Here's how the part is built. I have some questions about the finished solid (model axes, mm). A direction names the side the tool comes from. Round coordinates to 2 decimals unless told otherwise and drop trailing zeros. Order: outer loops, then holes, each group sorted by start corner. A loop starts at its lowest first (then second) coordinate and runs counter-clockwise, first axis right, second up. Notation, with made-up numbers: (22.25, 31) -> (39.25, 31) arc R13 ccw to (39.25, 52) -> close; hole circle Ø8 at (-20.75, 19.5). An arc over 180 degrees is marked (long way). Use a Markdown table: item, result. Add a question column.
from build123d import *

# Parameters (mm, degrees)
F0_W     = 60
F0_H     = 120
F1_DEPTH = 60
F2_R     = 3
F3_DEPTH = 7
F4_R     = 20
F5_R     = 10
F6_R     = 23.5
F7_DEPTH = 10
F8_W     = 30
F8_H     = 25
F9_DEPTH = 3


with BuildPart() as f1:
    # F0 (on Top) → F1 (new body)
    with BuildSketch(Plane.XY):
        Rectangle(F0_W, F0_H)
    extrude(amount=F1_DEPTH)

    # F2 (on face) → F3 (cut)
    with BuildSketch(Plane(origin=(0, 0, 0), x_dir=(1, 0, 0), z_dir=(0, 0, -1))):
        with Locations((5, -30)):
            Circle(F2_R)
    extrude(amount=-F3_DEPTH, mode=Mode.SUBTRACT)

    # F4
    f4_edges = [f1.edges().sort_by_distance(p)[0] for p in [
        (30, 0, 60),
        (-30, 0, 60),
    ]]
    fillet(f4_edges, radius=F4_R)

    # F5
    f5_edges = [f1.edges().sort_by_distance(p)[0] for p in [
        (30, 0, 0),
        (-30, 0, 0),
    ]]
    fillet(f5_edges, radius=F5_R)

    # F6 (on face) → F7 (join)
    with BuildSketch(Plane(origin=(0, 60, 0), x_dir=(-1, 0, 0), z_dir=(0, 1, 0))):
        with Locations((-5, 31.7827425897)):
            Circle(F6_R)
    extrude(amount=F7_DEPTH)

    # F8 (on face) → F9 (cut)
    with BuildSketch(Plane(origin=(0, 0, 0), x_dir=(1, 0, 0), z_dir=(0, 0, -1))):
        with Locations((5, 47.5)):
            Rectangle(F8_W, F8_H)
    extrude(amount=-F9_DEPTH, mode=Mode.SUBTRACT)


solid = f1.part
(1) I'm going to push flat-ended pins straight in: P1, Ø10, axis at y = -9, z = 51.5, coming from the +X side; P2, Ø2.5, axis at y = -51, z = 2, coming from the -X side; P3, Ø7.5, axis at x = 5.5, y = -46.5, coming from the -Z side. Where does each tip first touch, or does it pass through?
(2) If we mould it in two halves opening along Y, with no side actions, what happens to faces 5 (the flat face through (5, 70, 32)), 6 (the cylindrical face through (2.6, 31.8, 3.5)), 7 (the cylindrical face through (26.99, 0.84, 2.85)), 8 (the flat face through (5, -35, 1))? For each: pulls with the +Y half, pulls with the -Y half, needs draft (parallel to the pull), parting line crosses it, or undercut.
(3) Please list where these lines run through material, in increasing order: probe 1 along Y at (x, z) = (5, 4.75); probe 2 along Y at (x, z) = (-6, 6); probe 3 along Y at (x, z) = (5, 2). Write a range as from..to.
(4) I want a section at C-C on z = 33.5. List the corners of the cut face in (x, y) for me, and give its area (3 significant figures).
(5) I want a section at D-D on y = 1. List the corners of the cut face in (x, z) for me.
(6) On a 3-axis mill with a long thin cutter (end or side, diameter ignored), from which of +Z, -Z, +X, -X, +Y, -Y can I reach the whole of each face in a straight line? I mean faces 1 (the flat face through (5, 30, 7)), 2 (the flat face through (30, -1, 25)), 3 (the cylindrical face through (-5.84, 64.93, 10.93)), 4 (the flat face through (-10, -47, 1)). Say none if no direction works.
(7) I want a section at B-B on y = 30. List the corners of the cut face in (x, z) for me, and give its area (3 significant figures).
(8) I want a section at A-A on x = 5. List the corners of the cut face in (y, z) for me.
Output:
| question | item | result |
|---|---|---|
| 1 | P1 | x = 28.91 |
| 1 | P2 | x = -27.38 |
| 1 | P3 | z = 3 |
| 2 | face 5 | pulls with the +Y half |
| 2 | face 6 | undercut |
| 2 | face 7 | needs draft |
| 2 | face 8 | pulls with the -Y half |
| 3 | probe 1 | -60..27, 33..60 |
| 3 | probe 2 | -60..60 |
| 3 | probe 3 | -35..27, 33..60 |
| 4 | outline | (-30, -60) -> (30, -60) -> (30, 60) -> (28.44, 60) -> (28.44, 70) -> (-18.44, 70) -> (-18.44, 60) -> (-30, 60) -> close |
| 4 | area | 7,670 mm² |
| 5 | outline | (-30, 10) arc R10 ccw to (-20, 0) -> (20, 0) arc R10 ccw to (30, 10) -> (30, 40) arc R20 ccw to (10, 60) -> (-10, 60) arc R20 ccw to (-30, 40) -> close |
| 6 | face 1 | -Z |
| 6 | face 2 | +Z, -Z, +X, +Y, -Y |
| 6 | face 3 | +Y |
| 6 | face 4 | -Z, -Y |
| 7 | outline | (-30, 10) arc R10 ccw to (-20, 0) -> (2, 0) -> (2, 7) -> (8, 7) -> (8, 0) -> (20, 0) arc R10 ccw to (30, 10) -> (30, 40) arc R20 ccw to (10, 60) -> (-10, 60) arc R20 ccw to (-30, 40) -> close |
| 7 | area | 3,340 mm² |
| 8 | outline | (-60, 3) -> (-35, 3) -> (-35, 0) -> (27, 0) -> (27, 7) -> (33, 7) -> (33, 0) -> (60, 0) -> (60, 8.28) -> (70, 8.28) -> (70, 55.28) -> (60, 55.28) -> (60, 60) -> (-60, 60) -> close |
